Work out the finished part from the listing and answer in its coordinate system (mm). A direction names the side the tool comes from. Give positions to 0.01 mm unless a question says otherwise; leave off trailing zeros. Order: outer loops, then holes, each group sorted by start corner. A loop starts at its lowest first (then second) coordinate and runs counter-clockwise, first axis right, second up. Notation, with made-up numbers: (19.25, 86) - (46.25, 86) arc R38 cw to (46.25, 125) - close; hole circle Ø7 at (9, 35). An arc over 180 degrees is marked (long way). Put each result on its own line as item: value.
Autodesk Inventor part; units mm, degrees
ref_plane "YZ Plane" through (0, 0, 0) normal (1, 0, 0) x (0, 1, 0)
ref_plane "XZ Plane" through (0, 0, 0) normal (0, 1, 0) x (-1, 0, 0)
ref_plane "XY Plane" through (0, 0, 0) normal (0, 0, 1) x (1, 0, 0)
sketch "スケッチ1" plane through (0, 0, 0) normal (1, 0, 0) x (0, 1, 0)
  arc A0 (-5.655, 32.8818) -> (6.5548, 35.3105) centre (5.6756, 7.8246) ccw
  circle A1 centre (5.6756, -1.1754) radius 1.7
  circle A2 centre (5.6756, 16.8246) radius 1.7
  circle A3 centre (5.6756, 7.8246) radius 5.2
  line L0 (-1.6304, 24.0509) -> (-5.655, 32.8818)
  line L1 (6.5548, 35.3105) -> (6.2159, 25.6116)
  line L2 (6.2159, 25.6116) -> (-1.6304, 24.0509)
  point P0 (0, 0)
extrude "押し出し1" add sketch "スケッチ1" along normal blind 2.5
properties part number "belt_liner_v2_3DP_P-1-F" material "ABS プラスチック"
(1) Section D-D, the plane y = -16 is taken. Write down the section's boundary in (x, z).
Geometry check:
outline: (0, -9.1) - (2.5, -9.1) - (2.5, 24.75) - (0, 24.75) - close
(2) Section C-C, the plane z = 30.5 is taken. Write down the section's boundary in (x, y).
Geometry check:
outline: (0, -9.88) - (2.5, -9.88) - (2.5, -4.57) - (0, -4.57) - close; (0, 6.39) - (2.5, 6.39) - (2.5, 21.23) - (0, 21.23) - close
(3) A tool of negligible diameter and unlimited length cuts with its end or side. For faces 5 (the face through (1.232, -3.615, 28.405)), 6 (the face through (1.232, 7.246, -0.524)), from which of +Z, -Z, +X, -X, +Y, -Y can it reach the whole face along a straight path? Write none if from no direction.
Geometry check:
face 5: +Z, +X, -X
face 6: +X, -X
(4) Section A-A, the plane z = 17.5 is taken. Write down the section's boundary in (x, y).
Geometry check:
outline: (0, -20.07) - (2.5, -20.07) - (2.5, 4.12) - (0, 4.12) - close; (0, 7.24) - (2.5, 7.24) - (2.5, 31.42) - (0, 31.42) - close
(5) Straight lines are drawn through the part: line 1 (Y direction, x = 1.9, z = 5.5); line 2 (Y direction, x = 0.3, z = 5); line 3 (Z direction, x = 0.35, y = 7). For each, find the intervals that lie inside material, in ascending order.
Geometry check:
line 1: y = -21.73 to 1.02, 10.33 to 33.08
line 2: y = -21.68 to 1.31, 10.04 to 33.03
line 3: z = -19.64 to -2.24, -0.11 to 2.8, 12.85 to 15.76, 17.89 to 35.29
(6) Given pin 1 (3 mm diameter, centred on y = 5.68, z = -1.18, fed in from -X), flat-ended and moving along its own axis, determine where the tip first touches the part or whether it passes through.
Geometry check:
pin 1: passes through
(7) Section B-B, the plane x = 1.85 is taken. Write down the section's boundary in (y, z) (1 decimal).
Geometry check:
outline: (-5.7, 32.9) arc R27.5 ccw (long way) to (6.6, 35.3) - (6.2, 25.6) - (-1.6, 24.1) - close; hole circle Ø10.4 at (5.7, 7.8); hole circle Ø3.4 at (5.7, -1.2); hole circle Ø3.4 at (5.7, 16.8)
(8) Determine the mould class of faces 1 (the face through (1.232, 5.307, 18.484)), 2 (the face through (1.232, 12.136, -18.906)), 3 (the face through (1.232, 2.348, 24.842)), 4 (the face through (0, 5, 2)) for opening direction Z: pulls with the +Z half, pulls with the -Z half, needs draft (parallel to the pull), parting line crosses it, or undercut.
Geometry check:
face 1: undercut
face 2: parting line crosses it
face 3: pulls with the +Z half
face 4: needs draft
